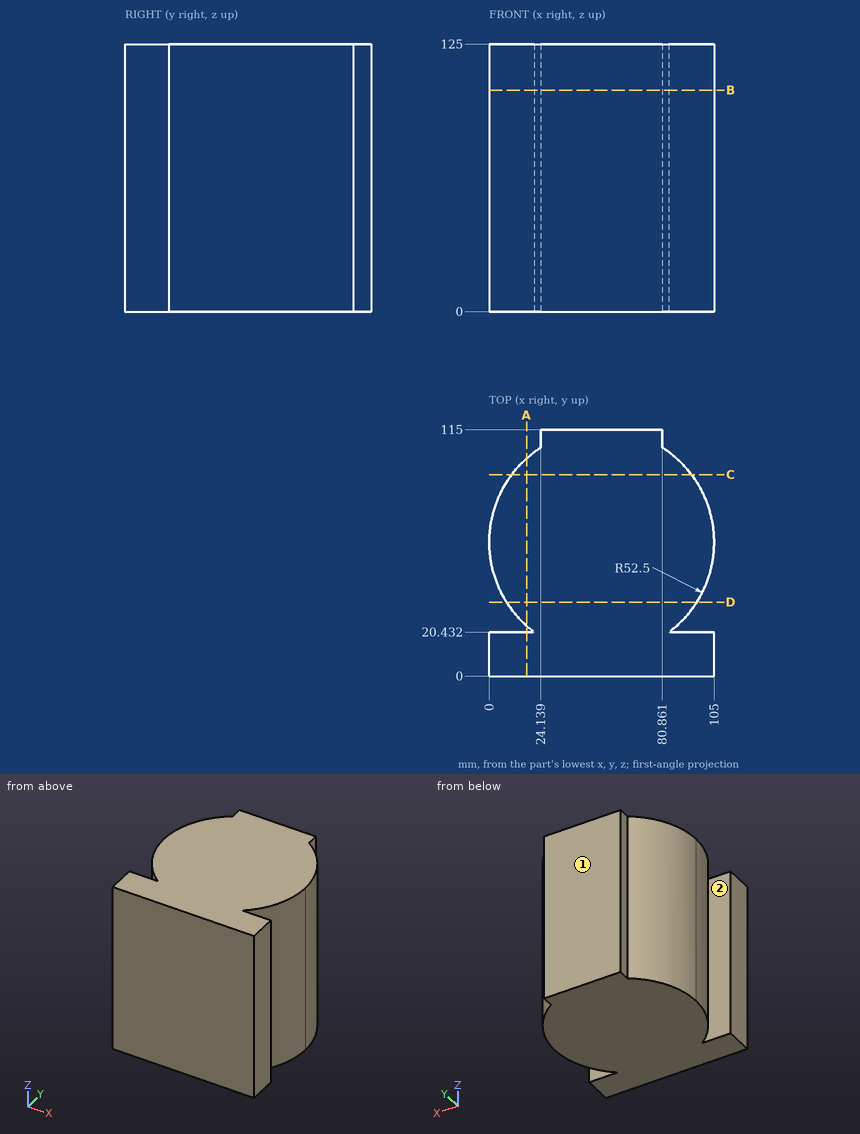
Can you work these out from the drawing? Everything is in mm from the part's minimum corner. A direction names the side the tool comes from. Give positions to 0.01 mm unless a question says otherwise; leave off trailing zeros. Loops run counter-clockwise (first coordinate to the right, second up) from the corner with the lowest first, then second, coordinate; pieces in that order, holes last. Notation, with made-up numbers: (80.5, 36) -> (113.5, 36) arc R28 ccw to (113.5, 66) -> close; hole circle Ø8 at (-35, -35). An arc over 180 degrees is marked (long way). Return JSON: item names as keys, results as strings.
Q1. I want a section at B-B, the plane z = 103.5. List the corners of the cut face in (x, y) for me.
Checks:
{"outline": "(0, 0) -> (105, 0) -> (105, 20.43) -> (83.91, 20.43) arc R52.5 ccw to (80.86, 106.68) -> (80.86, 115) -> (24.14, 115) -> (24.14, 106.68) arc R52.5 ccw to (21.09, 20.43) -> (0, 20.43) -> close"}
Q2. I want a section at C-C, the plane y = 94. List the corners of the cut face in (x, z) for me.
Checks:
{"outline": "(10.5, 0) -> (94.5, 0) -> (94.5, 125) -> (10.5, 125) -> close"}
Q3. I want a section at D-D, the plane y = 34.5. List the corners of the cut face in (x, z) for me.
Checks:
{"outline": "(8.09, 0) -> (96.91, 0) -> (96.91, 125) -> (8.09, 125) -> close"}
Q4. For pin 1 Ø5 at (y, z) = (85.5, 53.5) entering from +X; pin 2 Ø6.5 at (x, z) = (11, 46.5) entering from +Y; pin 3 Ø4 at (y, z) = (112, 76) entering from -X, each with a flat end and sliding along its axis, tell me the tip position at first contact or that it passes through.
Checks:
{"pin 1": "stops at x = 100.83", "pin 2": "stops at y = 98.46", "pin 3": "stops at x = 24.14"}
Q5. I need wall thicknesses on probe 1 along Y at (x, z) = (19, 34) (1 decimal); probe 2 along Y at (x, z) = (6, 66) (1 decimal); probe 3 along X at (y, z) = (110, 112.5). Which ranges of each line are inside material? Lowest first, please.
Checks:
{"probe 1": "y = 0 to 20.4, 22.1 to 102.9", "probe 2": "y = 0 to 20.4, 38.1 to 86.9", "probe 3": "x = 24.14 to 80.86"}
Q6. On a 3-axis mill with a long thin cutter (end or side, diameter ignored), from which of +Z, -Z, +X, -X, +Y, -Y can I reach the whole of each face in a straight line? I mean the marked faces 1 and 2. Say none if no direction works.
Checks:
{"face 1": "+Z, -Z, +X, -X, +Y", "face 2": "+Z, -Z, -X"}
Q7. I want a section at A-A, the plane x = 17.5. List the corners of the cut face in (y, z) for me.
Checks:
{"outline": "(0, 0) -> (20.43, 0) -> (20.43, 125) -> (0, 125) -> close; (23.37, 0) -> (101.63, 0) -> (101.63, 125) -> (23.37, 125) -> close"}
